Geometry: final body of the model. Coordinates: model frame, mm. Face numbers are marked on the shaded views. A direction names the side the tool comes from. Give positions to 0.01 mm unless a question says otherwise; leave off trailing zeros. Write each loop counter-clockwise with the first axis right and the second up, starting at its lowest first coordinate (ties: lowest second). Pieces come first, ordered by that corner, then holes.
Q1. Cut plane A-A on z = 0. Return the cut outline in (x, y).
Q2. Line query: L1, parallel to X at y = 4.2, z = 0; L2, parallel to X at y = 1.5, z = -5.5; L3, parallel to X at y = 2.75, z = 9.5. Output: solid intervals per line, ascending.
Q3. Cut plane C-C on y = 5.25. Return the cut outline in (x, z).
Q4. Reachability of the marked faces 4, 5 and 6 from +Z, -Z, +X, -X, +Y, -Y: full face, straight path, thin tool, end or side. Return the list, or none.
Q5. Cut plane D-D on x = -12. Return the cut outline in (y, z).
Q6. Cut plane B-B on x = 0. Return the cut outline in (y, z).
Q7. Pin query (flat end, axial travel): pin 1 (1 mm diameter, centred on y = 5, z = -7, fed in from +X); pin 2 (1.8 mm diameter, centred on x = 5.64, z = 5.67, fed in from +Y); pin 3 (3 mm diameter, centred on y = 3, z = -11, fed in from -X); pin 4 (4 mm diameter, centred on x = 0, z = 0, fed in from +Y). Return the tip coordinate at first contact, or that it passes through.
Q8. Draft query along Z for the marked faces 1, 2 and 3. Return one class per face: pulls with the +Z half, pulls with the -Z half, needs draft (parallel to the pull), parting line crosses it, or undercut.
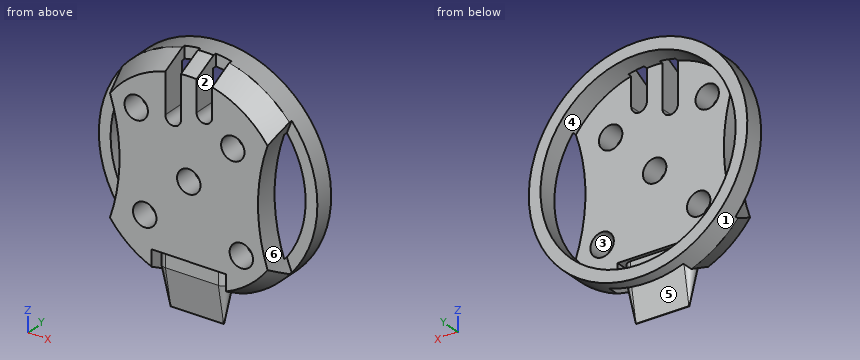
```python
from build123d import *
from OCP.BRepFilletAPI import BRepFilletAPI_MakeChamfer

# Parameters (mm, degrees)
SCHIZZO1_R                   = 14
ESTRUSIONE_ESTRUSIONE1_DEPTH = 6
SCHIZZO2_W                   = 9.5
SCHIZZO2_H                   = 5
TAGLIO_ESTRUSIONE1_DEPTH     = 4.5
SCHIZZO3_R                   = 12.5
TAGLIO_ESTRUSIONE2_DEPTH     = 3
TAGLIO_ESTRUSIONE4_DEPTH     = 3.5
SMUSSO1_SIZE                 = 1.5
SMUSSO1_SIZE2                = 3.075455762
SCHIZZO8_R                   = 22.778601144
TAGLIO_ESTRUSIONE6_DEPTH     = 3.5
ESTRUSIONE_ESTRUSIONE2_DEPTH = 7
SMUSSO2_SIZE                 = 5
SMUSSO2_SIZE2                = 0.971901546
SCHIZZO14_R                  = 1.5
TAGLIO_ESTRUSIONE10_DEPTH    = 23.455511573
SCHIZZO17_R                  = 1.5
TAGLIO_ESTRUSIONE12_DEPTH    = 32


with BuildPart() as part:
    # Schizzo1 → Estrusione-Estrusione1 (new body)
    with BuildSketch(Plane(origin=(0, 0, 0), x_dir=(1, 0, 0), z_dir=(0, 1, 0))):
        with Locations(Location((0, 0, 0), (0, 0, 270))):
            Circle(SCHIZZO1_R)
    extrude(amount=ESTRUSIONE_ESTRUSIONE1_DEPTH)

    # Schizzo2 → Taglio-Estrusione1 (cut)
    with BuildSketch(Plane.XZ):
        with Locations((0, -12)):
            Rectangle(SCHIZZO2_W, SCHIZZO2_H)
    extrude(amount=-TAGLIO_ESTRUSIONE1_DEPTH, mode=Mode.SUBTRACT)

    # Schizzo3 → Taglio-Estrusione2 (cut)
    with BuildSketch(Plane(origin=(0, 6, 0), x_dir=(1, 0, 0), z_dir=(0, 1, 0))):
        with Locations(Location((0, 0, 0), (0, 0, 270))):
            Circle(SCHIZZO3_R)
    extrude(amount=-TAGLIO_ESTRUSIONE2_DEPTH, mode=Mode.SUBTRACT)

    # Schizzo4 → Taglio-Estrusione4 (cut)
    with BuildSketch(Plane.XZ):
        with BuildLine():
            Line((-1, 7), (-1, 13.964240044))
            ThreePointArc((-1, 13.964240044), (-2.00522934, 13.855650663), (-3, 13.674794331))
            Line((-3, 13.674794331), (-3, 7))
            ThreePointArc((-3, 7), (-2, 6), (-1, 7))
        make_face()
        with BuildLine():
            ThreePointArc((3, 13.674794331), (2.00522934, 13.855650663), (1, 13.964240044))
            Line((1, 13.964240044), (1, 8.5))
            ThreePointArc((1, 8.5), (2, 7.5), (3, 8.5))
            Line((3, 8.5), (3, 13.674794331))
        make_face()
    extrude(amount=-TAGLIO_ESTRUSIONE4_DEPTH, mode=Mode.SUBTRACT)

    # Smusso1
    smusso1_edges = [part.edges().sort_by_distance(p)[0] for p in [
        (0.500319591, 0, 13.991057155),
        (-13.970345786, 0, 0.910735206),
        (13.970345786, 0, 0.910735206),
    ]]
    smusso1_side = [part.faces().sort_by_distance(p)[0] for p in [
        (0.010947271, 0, 0.331138895),
    ]]
    chamfer(smusso1_edges, length=SMUSSO1_SIZE, length2=SMUSSO1_SIZE2, reference=smusso1_side[0])

    # Schizzo8 → Taglio-Estrusione6 (cut)
    with BuildSketch(Plane.XZ):
        with Locations((-31.649021425, 0)):
            Circle(SCHIZZO8_R)
        with Locations((31.649021425, 0)):
            Circle(SCHIZZO8_R)
    extrude(amount=-TAGLIO_ESTRUSIONE6_DEPTH, mode=Mode.SUBTRACT)

    # Schizzo10 → Estrusione-Estrusione2 (add)
    with BuildSketch(Plane(origin=(0, 0, -9.5), x_dir=(-1, 0, 0), z_dir=(0, 0, -1))):
        with BuildLine():
            Line((-3.389234254, 2.559575442), (3.389234254, 2.559575442))
            ThreePointArc((3.389234254, 2.559575442), (4.389234254, 1.559575442), (3.389234254, 0.559575442))
            Line((3.389234254, 0.559575442), (-3.389234254, 0.559575442))
            ThreePointArc((-3.389234254, 0.559575442), (-4.389234254, 1.559575442), (-3.389234254, 2.559575442))
        make_face()
    extrude(amount=ESTRUSIONE_ESTRUSIONE2_DEPTH)

    # Smusso2: one chamfer whose edges measure the first distance from different faces: ONE call of the kernel's chamfer builder (chamfer() names one face for all edges)
    smusso2_edges_1 = [part.edges().sort_by_distance(p)[0] for p in [
        (4.389234254, 1.559575442, -16.5),
    ]]
    smusso2_side_1 = [part.faces().sort_by_distance(p)[0] for p in [
        (4.389234254, 1.559575442, -13),
    ]]
    smusso2_edges_2 = [part.edges().sort_by_distance(p)[0] for p in [
        (0, 0.559575442, -16.5),
    ]]
    smusso2_side_2 = [part.faces().sort_by_distance(p)[0] for p in [
        (0, 0.559575442, -13),
    ]]
    smusso2_edges_3 = [part.edges().sort_by_distance(p)[0] for p in [
        (-4.389234254, 1.559575442, -16.5),
    ]]
    smusso2_side_3 = [part.faces().sort_by_distance(p)[0] for p in [
        (-4.389234254, 1.559575442, -13),
    ]]
    smusso2_edges_4 = [part.edges().sort_by_distance(p)[0] for p in [
        (0, 2.559575442, -16.5),
    ]]
    smusso2_side_4 = [part.faces().sort_by_distance(p)[0] for p in [
        (0, 2.559575442, -13),
    ]]
    smusso2 = BRepFilletAPI_MakeChamfer(part.part.solid().wrapped)
    for e in smusso2_edges_1:
        smusso2.Add(SMUSSO2_SIZE, SMUSSO2_SIZE2, e.wrapped, smusso2_side_1[0].wrapped)  # the first distance lies on this face
    for e in smusso2_edges_2:
        smusso2.Add(SMUSSO2_SIZE, SMUSSO2_SIZE2, e.wrapped, smusso2_side_2[0].wrapped)  # the first distance lies on this face
    for e in smusso2_edges_3:
        smusso2.Add(SMUSSO2_SIZE, SMUSSO2_SIZE2, e.wrapped, smusso2_side_3[0].wrapped)  # the first distance lies on this face
    for e in smusso2_edges_4:
        smusso2.Add(SMUSSO2_SIZE, SMUSSO2_SIZE2, e.wrapped, smusso2_side_4[0].wrapped)  # the first distance lies on this face
    add(Compound.cast(smusso2.Shape()), mode=Mode.REPLACE)

    # Schizzo14 → Taglio-Estrusione10 (cut, through all)
    with BuildSketch(Plane.XZ):
        with Locations(Location((6.733876165, -6.701112728, 0), (0, 0, 270))):
            Circle(SCHIZZO14_R)
        with Locations(Location((-6.733876165, 6.701112728, 0), (0, 0, 270))):
            Circle(SCHIZZO14_R)
        with Locations(Location((5.643042298, 5.67063256, 0), (0, 0, 270))):
            Circle(SCHIZZO14_R)
        with Locations(Location((-5.643042298, -5.67063256, 0), (0, 0, 270))):
            Circle(SCHIZZO14_R)
    extrude(amount=-TAGLIO_ESTRUSIONE10_DEPTH, mode=Mode.SUBTRACT)

    # Schizzo17 → Taglio-Estrusione12 (cut)
    with BuildSketch(Plane.XZ):
        with Locations(Location((0, 0, 0), (0, 0, 270))):
            Circle(SCHIZZO17_R)
    extrude(amount=-TAGLIO_ESTRUSIONE12_DEPTH, mode=Mode.SUBTRACT)


solid = part.part
```
Data:
1. outline: (-14, 3.5) - (-12.5, 3.5) - (-12.5, 6) - (-14, 6) - close; (-8.87, 0) - (-1.5, 0) - (-1.5, 3) - (-8.87, 3) - close; (1.5, 0) - (8.87, 0) - (8.87, 3) - (1.5, 3) - close; (12.5, 3.5) - (14, 3.5) - (14, 6) - (12.5, 6) - close
2. L1: x = -14 to -12.5, 12.5 to 14
2. L2: x = -9.54 to -7.13, -4.15 to 5.84, 7.63 to 9.54
2. L3: x = -10.07 to -3, -1 to 1, 3 to 10.07
3. outline: circle Ø28 at (0, 0); hole circle Ø25 at (0, 0)
4. face 4: +Y
4. face 5: -Z
4. face 6: +X, -Y
5. outline: (3.5, -7.21) - (6, -7.21) - (6, -3.5) - (3.5, -3.5) - close; (3.5, 3.5) - (6, 3.5) - (6, 7.21) - (3.5, 7.21) - close
6. outline: (0, -9.5) - (0.56, -9.5) - (0.56, -11.5) - (1.53, -16.5) - (1.59, -16.5) - (2.56, -11.5) - (2.56, -9.5) - (3, -9.5) - (3, -1.5) - (0, -1.5) - close; (0, 1.5) - (3, 1.5) - (3, 12.5) - (6, 12.5) - (6, 14) - (3.08, 14) - (0, 12.5) - close; (4.5, -14) - (6, -14) - (6, -12.5) - (4.5, -12.5) - close
7. pin 1: stops at x = 12.4
7. pin 2: passes through
7. pin 3: stops at x = -10.28
7. pin 4: stops at y = 3
8. face 1: parting line crosses it
8. face 2: needs draft
8. face 3: undercut
